Read the model definition and answer for the solid it produces. Units are mm, in the model's axes. A direction names the side the tool comes from. Coordinates: 2 decimals unless noted, no trailing zeros. Order: outer loops, then holes, each group sorted by start corner. A loop starts at its lowest first (then second) coordinate and runs counter-clockwise, first axis right, second up. Notation, with made-up numbers: M 10,13.5 L 16,13.5 A27 cw 16,44.5 Z; hole C -17.5,34.5 d10. An arc over 180 degrees is marked long. Put each result on its own line as item: value.
from build123d import *

# Parameters (mm, degrees)
F1_DEPTH = 4


with BuildPart() as f1:
    # F0 (on Top) → F1 (new body)
    with BuildSketch(Plane.XY):
        Polygon((116.286797, -137.5), (137.5, -137.5), (137.5, -116.286797), (133.713203, -112.5), (112.5, -112.5), (112.5, -133.713203), align=None)
        with BuildLine():
            ThreePointArc((129, -125), (128.695518, -126.530734), (127.828427, -127.828427))
            ThreePointArc((127.828427, -127.828427), (121.304482, -123.469266), (129, -125))
        make_face(mode=Mode.SUBTRACT)
        Polygon((78.786797, -100), (112.5, -133.713203), (112.5, -112.5), (133.713203, -112.5), (100, -78.786797), (100, -100), align=None)
        Polygon((-78.786797, -100), (78.786797, -100), (100, -100), (100, -78.786797), (100, 78.786797), (100, 100), (78.786797, 100), (-78.786797, 100), (-100, 100), (-100, 78.786797), (-100, -78.786797), (-100, -100), align=None)
        Polygon((-112.5, -133.713203), (-78.786797, -100), (-100, -100), (-100, -78.786797), (-133.713203, -112.5), (-112.5, -112.5), align=None)
        Polygon((100, 100), (100, 78.786797), (133.713203, 112.5), (112.5, 112.5), (112.5, 133.713203), (78.786797, 100), align=None)
        Polygon((-116.286797, -137.5), (-112.5, -133.713203), (-112.5, -112.5), (-133.713203, -112.5), (-137.5, -116.286797), (-137.5, -137.5), align=None)
        with BuildLine():
            ThreePointArc((-121, -125), (-123.469266, -128.695518), (-127.828427, -127.828427))
            ThreePointArc((-127.828427, -127.828427), (-126.530734, -121.304482), (-121, -125))
        make_face(mode=Mode.SUBTRACT)
        Polygon((112.5, 112.5), (133.713203, 112.5), (137.5, 116.286797), (137.5, 137.5), (116.286797, 137.5), (112.5, 133.713203), align=None)
        with BuildLine():
            ThreePointArc((129, 125), (121.304482, 123.469266), (127.828427, 127.828427))
            ThreePointArc((127.828427, 127.828427), (128.695518, 126.530734), (129, 125))
        make_face(mode=Mode.SUBTRACT)
        Polygon((-133.713203, 112.5), (-100, 78.786797), (-100, 100), (-78.786797, 100), (-112.5, 133.713203), (-112.5, 112.5), align=None)
        Polygon((-137.5, 116.286797), (-133.713203, 112.5), (-112.5, 112.5), (-112.5, 133.713203), (-116.286797, 137.5), (-137.5, 137.5), align=None)
        with BuildLine():
            ThreePointArc((-121, 125), (-126.530734, 121.304482), (-127.828427, 127.828427))
            ThreePointArc((-127.828427, 127.828427), (-123.469266, 128.695518), (-121, 125))
        make_face(mode=Mode.SUBTRACT)
    extrude(amount=F1_DEPTH)


solid = f1.part
Q1. A tool of negligible diameter and unlimited length cuts with its end or side. For faces 4 (the face through (119.012, -97.799, 1.972)), 5 (the face through (97.799, 119.012, 1.972)), 6 (the face through (97.274, -118.488, 1.972)), from which of +Z, -Z, +X, -X, +Y, -Y can it reach the whole face along a straight path? Write none if from no direction.
Answers below:
face 4: +Z, -Z, +X
face 5: +Z, -Z, +Y
face 6: +Z, -Z, -Y
Q2. Find section B-B on y = -18. Write down the section's boundary in (x, z), plus the area to 3 significant figures.
Answers below:
outline: M -100,0 L 100,0 L 100,4 L -100,4 Z
area: 800 mm^2
Q3. Find section A-A on z = 2.2. Write down the section's boundary in (x, y).
Answers below:
outline: M -137.5,-137.5 L -116.29,-137.5 L -78.79,-100 L 78.79,-100 L 116.29,-137.5 L 137.5,-137.5 L 137.5,-116.29 L 100,-78.79 L 100,78.79 L 137.5,116.29 L 137.5,137.5 L 116.29,137.5 L 78.79,100 L -78.79,100 L -116.29,137.5 L -137.5,137.5 L -137.5,116.29 L -100,78.79 L -100,-78.79 L -137.5,-116.29 Z; hole C -125,-125 d8; hole C -125,125 d8; hole C 125,-125 d8; hole C 125,125 d8
Q4. For a pull along X with two mould halves and no side action, classify faces 1 (the face through (118.488, 97.274, 1.972)), 2 (the face through (-119.012, 97.799, 1.972)), 3 (the face through (-97.799, -119.012, 1.972)) as +X half, -X half, draft (parallel to the pull), parting line (faces both ways), or undercut.
Answers below:
face 1: +X half
face 2: -X half
face 3: undercut
Q5. Consider line 1 along Y through (x, z) = (-125, 2); line 2 along X through (y, z) = (-18, 0.7). Determine where each line is inside the solid, lowest interval first.
Answers below:
line 1: y = -137.5 to -129, -121 to -103.79, 103.79 to 121, 129 to 137.5
line 2: x = -100 to 100
Q6. Given pin 1 (1.2 mm diameter, centred on x = 3.5, z = 1, fed in from +Y); pin 2 (1.2 mm diameter, centred on y = 28.5, z = 2.5, fed in from +X); pin 3 (1.5 mm diameter, centred on x = 99.5, z = 2.5, fed in from +Y); pin 4 (7 mm diameter, centred on x = 125, y = -125, fed in from -Z), each flat-ended and moving along its own axis, determine where each tip first touches the part or whether it passes through.
Answers below:
pin 1: stops at y = 100
pin 2: stops at x = 100
pin 3: stops at y = 121.46
pin 4: passes through
